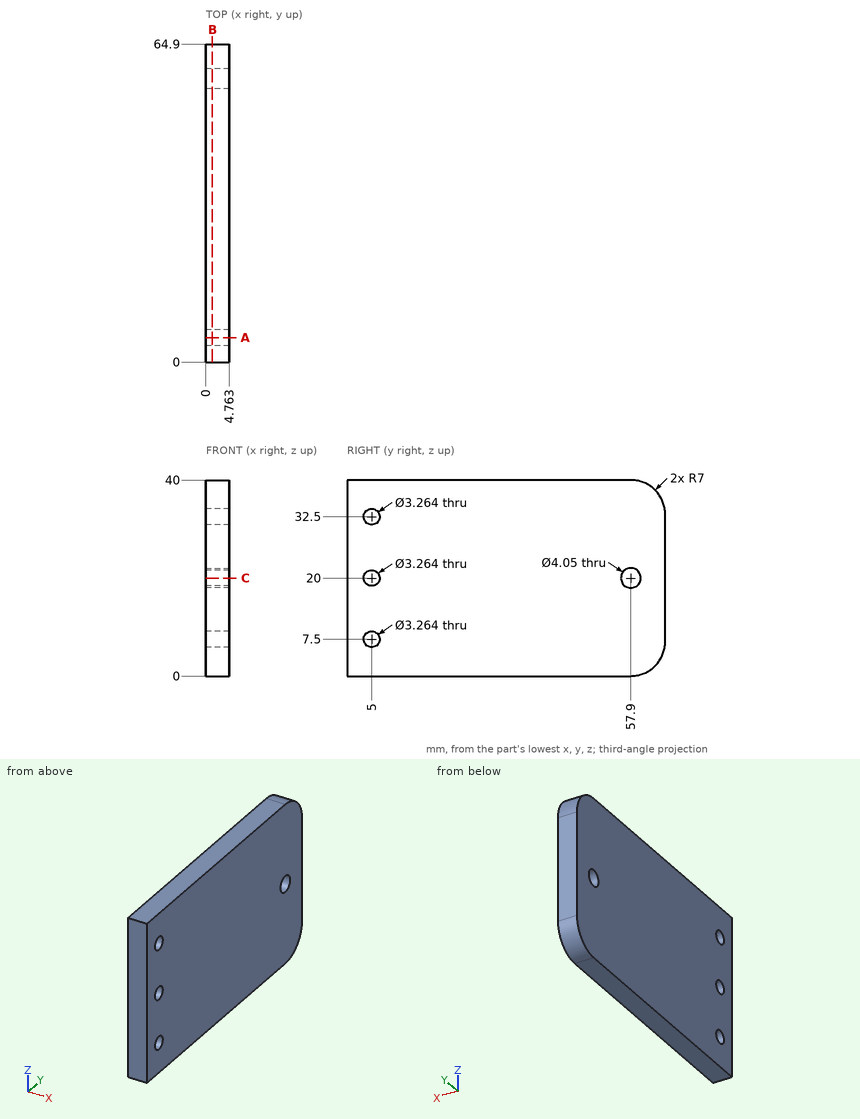
Geometry: see drawing. Coordinates: mm, zero at the bounding-box minimum. Give positions to 0.01 mm unless a question says otherwise; leave off trailing zeros. Write each loop counter-clockwise with the first axis right and the second up, starting at its lowest first coordinate (ties: lowest second). Pieces come first, ordered by that corner, then holes. Notation, with made-up numbers: (52, 41.5) - (75, 41.5) arc R34 cw to (75, 71.5) - close; hole circle Ø6 at (46, 72.5). An arc over 180 degrees is marked (long way). Return JSON: item names as keys, results as strings. Group by question number.
1) Line query: line 1 (Y direction, x = 2.45, z = 20) (1 decimal); line 2 (Y direction, x = 2.25, z = 7.5); line 3 (Y direction, x = 2.2, z = 9) (1 decimal). Output: solid intervals per line, ascending.
2) Section A-A on y = 5. Return the cut outline in (x, z).
3) Section C-C on z = 20. Return the cut outline in (x, y) (1 decimal), plus the area to 3 significant figures.
4) Section B-B on x = 1.35. State how many separate pieces and enclosed holes the cut face has, plus the area to 3 significant figures.
Filled in:
{
 "1": {"line 1": "y = 0 to 3.4, 6.6 to 55.9, 59.9 to 64.9", "line 2": "y = 0 to 3.37, 6.63 to 64.9", "line 3": "y = 0 to 4.4, 5.6 to 64.9"},
 "2": {"outline": "(0, 0) - (4.76, 0) - (4.76, 5.87) - (0, 5.87) - close; (0, 9.13) - (4.76, 9.13) - (4.76, 18.37) - (0, 18.37) - close; (0, 21.63) - (4.76, 21.63) - (4.76, 30.87) - (0, 30.87) - close; (0, 34.13) - (4.76, 34.13) - (4.76, 40) - (0, 40) - close"},
 "3": {"outline": "(0, 0) - (4.8, 0) - (4.8, 3.4) - (0, 3.4) - close; (0, 6.6) - (4.8, 6.6) - (4.8, 55.9) - (0, 55.9) - close; (0, 59.9) - (4.8, 59.9) - (4.8, 64.9) - (0, 64.9) - close", "area": "274 mm^2"},
 "4": {"separate pieces": "1", "enclosed holes": "4", "area": "2,540 mm^2"}
}
